Check sheet for the modelled part. Datum: model origin and axes. Units: mm. A direction names the side the tool comes from. Give positions to 0.01 mm unless a question says otherwise; leave off trailing zeros. Write each loop counter-clockwise with the first axis right and the second up, starting at its lowest first coordinate (ties: lowest second). Pieces come first, ordered by that corner, then holes. Notation, with made-up numbers: M 8.25,-38.5 L 58.25,-38.5 A12 cw 58.25,-28.5 Z; hole C 26,-28 d7. An arc over 180 degrees is marked long. Use CSV: the item, a comma, the result in double quotes. Start each with the question number.
1. Scan lines: line 1 (Z direction, x = 4.5, y = 459); line 2 (Z direction, x = -10.5, y = 283.5). Record each from-to range of solid material in increasing order.
2. Cross-section at A-A, the plane y = 119.5. Enter the section's corners in (x, z).
3. Mould release check, pull along X, two halves, no side actions. Record for faces 1 (the face through (0, 250, -11.049)), 2 (the face through (-12.7, 250, 0)), 3 (the face through (-0.2, 0, -11.5)): +X half, -X half, draft (parallel to the pull), parting line (faces both ways), or undercut.
4. Depth check by flat-ended pin: P1, Ø5, axis at y = 253.85, z = 0.08, coming from the -X side. Enter the tip coordinate at first touch or a pass-through.
5. Access from +Z, -Z, +X, -X, +Y, -Y to the whole of each face (thin tool, end or side, straight path). Record for faces 4 (the face through (0, 250, 11.049)), 5 (the face through (0, 250, 12.7)).
from build123d import *

# Parameters (mm, degrees)
SKETCH1_W                  = 25.4
SKETCH1_H                  = 25.4
SKETCH1_W_2                = 22.098
SKETCH1_H_2                = 22.098
BOSS_EXTRUDE1_DEPTH        = 508
FILLET1_R                  = 1.27
F_1_0_228_DIAMETER_HOLE2_D = 5.7912
F_8_32_TAPPED_HOLE1_D      = 3.4544


with BuildPart() as part:
    # Sketch1 → Boss-Extrude1 (new body)
    with BuildSketch(Plane(origin=(0, 0, 0), x_dir=(1, 0, 0), z_dir=(0, 1, 0))):
        Rectangle(SKETCH1_W, SKETCH1_H)
        Rectangle(SKETCH1_W_2, SKETCH1_H_2, mode=Mode.SUBTRACT)
    extrude(amount=BOSS_EXTRUDE1_DEPTH)

    # Fillet1
    fillet1_edges = [part.edges().sort_by_distance(p)[0] for p in [
        (-11.049, 254, 11.049),
        (11.049, 254, 11.049),
        (11.049, 254, -11.049),
        (-11.049, 254, -11.049),
        (12.7, 254, 12.7),
        (-12.7, 254, 12.7),
        (-12.7, 254, -12.7),
        (12.7, 254, -12.7),
    ]]
    fillet(fillet1_edges, radius=FILLET1_R)

    # #1 (0.228) Diameter Hole2 (through all)
    with Locations(Plane.ZY.offset(12.7)):
        with Locations((0.1524, 469.9), (0.1524, 355.6), (0.0762, 253.8476), (0.1524, 152.0952), (0.1524, 37.7952)):
            Hole(F_1_0_228_DIAMETER_HOLE2_D / 2)

    # #8-32 Tapped Hole1 (through all)
    with Locations(Plane.XY.offset(12.7)):
        with Locations((0, 9.271), (0.103095802, 498.729)):
            Hole(F_8_32_TAPPED_HOLE1_D / 2)


solid = part.part
Worked answers:
1,line 1,"z = -12.7 to -11.05, 11.05 to 12.7"
1,line 2,"z = -12.7 to -10.82, 10.82 to 12.7"
2,outline,"M -12.7,-11.43 A1.27 ccw -11.43,-12.7 L 11.43,-12.7 A1.27 ccw 12.7,-11.43 L 12.7,11.43 A1.27 ccw 11.43,12.7 L -11.43,12.7 A1.27 ccw -12.7,11.43 Z; hole M -11.05,-9.78 A1.27 ccw -9.78,-11.05 L 9.78,-11.05 A1.27 ccw 11.05,-9.78 L 11.05,9.78 A1.27 ccw 9.78,11.05 L -9.78,11.05 A1.27 ccw -11.05,9.78 Z"
3,face 1,"undercut"
3,face 2,"-X half"
3,face 3,"draft"
4,P1,"passes through"
5,face 4,"+Y, -Y"
5,face 5,"+Z, +X, -X, +Y, -Y"
